Here's how the part is built. I have some questions about the finished solid (model axes, mm). A direction names the side the tool comes from. Give positions to 0.01 mm unless a question says otherwise; leave off trailing zeros. Write each loop counter-clockwise with the first axis right and the second up, starting at its lowest first coordinate (ties: lowest second). Pieces come first, ordered by that corner, then holes. Notation, with made-up numbers: (30.5, 24.25) - (35.5, 24.25) arc R11 ccw to (35.5, 36.25) - close; hole circle Ø11 at (84, -14.75). An arc over 180 degrees is marked (long way). Use a Markdown table: item, result.
```python
from build123d import *

# Parameters (mm, degrees)
SKETCH2_R                      = 6.35
BOSS_EXTRUDE1_DEPTH            = 127
SKETCH3_R                      = 6.35
BOSS_EXTRUDE2_DEPTH            = 25.4
F_6_0_204_DIAMETER_HOLE1_D     = 5.1816
F_6_0_204_DIAMETER_HOLE1_DEPTH = 12.7
F_6_0_204_DIAMETER_HOLE1_TIP   = 1.556709692


with BuildPart() as part:
    # Sketch2 → Boss-Extrude1 (new body)
    with BuildSketch(Plane(origin=(0, 0, 0), x_dir=(1, 0, 0), z_dir=(0, 1, 0))):
        with Locations(Location((0, 0, 0), (0, 0, 270))):
            Circle(SKETCH2_R)
    extrude(amount=BOSS_EXTRUDE1_DEPTH)

    # Sketch3 → Boss-Extrude2 (add)
    with BuildSketch(Plane.XY):
        with Locations((0, 101.646656128)):
            Circle(SKETCH3_R)
        with Locations((0, 25.353343872)):
            Circle(SKETCH3_R)
    extrude(amount=BOSS_EXTRUDE2_DEPTH)

    # #6 (0.204) Diameter Hole1
    with Locations(Plane.XY.offset(25.4)):
        with Locations((0, 101.646656128), (0, 25.353343872)):
            Hole(F_6_0_204_DIAMETER_HOLE1_D / 2, depth=F_6_0_204_DIAMETER_HOLE1_DEPTH)
            with Locations((0, 0, -(F_6_0_204_DIAMETER_HOLE1_DEPTH + F_6_0_204_DIAMETER_HOLE1_TIP / 2))):  # 118° drill point
                Cone(0, F_6_0_204_DIAMETER_HOLE1_D / 2, F_6_0_204_DIAMETER_HOLE1_TIP, mode=Mode.SUBTRACT)


solid = part.part
```
Item 1: For faces 4 (the cylindrical face through (0.279, 62.611, -6.344)), 5 (the cylindrical face through (0.337, 104.215, 18.961)), 6 (the flat face through (0, 0, 0)), which set-ups out of +Z, -Z, +X, -X, +Y, -Y let a thin tool reach every point of the face, with its end or its side?
Values:
| item | result |
|---|---|
| face 4 | none |
| face 5 | +Z |
| face 6 | +Z, -Z, +X, -X, -Y |
Item 2: Will these pins go through, and if not, where does the flat tip stop? pin 1 Ø1 at (x, y) = (0.5, 110.5) entering from +Z; pin 2 Ø6 at (x, y) = (0, 25.35) entering from +Z; pin 3 Ø3 at (x, z) = (2, 9) entering from -Y; pin 4 Ø4 at (x, z) = (4, 7.5) entering from -Y.
Values:
| item | result |
|---|---|
| pin 1 | stops at z = 6.35 |
| pin 2 | stops at z = 25.4 |
| pin 3 | stops at y = 19.02 |
| pin 4 | stops at y = 19.33 |
Item 3: Thinking about a two-plate mould opening in Y: for faces 1 (the cylindrical face through (0.562, 22.824, 18.961)), 2 (the flat face through (0, 127, 0)), 3 (the flat face through (-0.1, 98.9, 25.4)), which applies, +Y half, -Y half, draft (parallel to the pull), parting line (faces both ways), or undercut?
Values:
| item | result |
|---|---|
| face 1 | undercut |
| face 2 | +Y half |
| face 3 | draft |
Item 4: If we section it at C-C, the plane y = 65: Write out the boundary of the cut face in (x, z).
Values:
| item | result |
|---|---|
| outline | circle Ø12.7 at (0, 0) |
Item 5: If we section it at D-D, the plane y = 30: Write out the boundary of the cut face in (x, z), plus the area to 3 significant figures.
Values:
| item | result |
|---|---|
| outline | (-4.33, 4.65) arc R6.35 ccw (long way) to (4.33, 4.65) - (4.33, 25.4) - (-4.33, 25.4) - close |
| area | 296 mm2 |
Item 6: If we section it at A-A, the plane z = 2.5: Write out the boundary of the cut face in (x, y), plus the area to 3 significant figures.
Values:
| item | result |
|---|---|
| outline | (-5.84, 0) - (5.84, 0) - (5.84, 22.85) arc R6.35 ccw to (5.84, 27.85) - (5.84, 99.15) arc R6.35 ccw to (5.84, 104.15) - (5.84, 127) - (-5.84, 127) - (-5.84, 104.15) arc R6.35 ccw to (-5.84, 99.15) - (-5.84, 27.85) arc R6.35 ccw to (-5.84, 22.85) - close |
| area | 1,490 mm2 |
Item 7: If we section it at B-B, the plane z = 18.5: Write out the boundary of the cut face in (x, y).
Values:
| item | result |
|---|---|
| outline | circle Ø12.7 at (0, 25.35); circle Ø12.7 at (0, 101.65); hole circle Ø5.18 at (0, 25.35); hole circle Ø5.18 at (0, 101.65) |
Item 8: I need wall thicknesses on line 1 along Y through (x, z) = (0, 19); line 2 along Y through (x, z) = (1.75, 13); line 3 along X through (y, z) = (48.5, -0.5). Which ranges of each line are inside material? Lowest first, please. Write a range as [from, to].
Values:
| item | result |
|---|---|
| line 1 | y = [19, 22.76], [27.94, 31.7], [95.3, 99.06], [104.24, 108] |
| line 2 | y = [19.25, 23.44], [27.26, 31.46], [95.54, 99.74], [103.56, 107.75] |
| line 3 | x = [-6.33, 6.33] |
